from build123d import *

# Parameters (mm, degrees)
F0_W     = 228.6
F0_H     = 101.6
F0_R     = 22.225
F0_R_2   = 3.175
F1_DEPTH = 9.525
F2_DEPTH = 5.08


with BuildPart() as f1:
    # F0 (on Top) → F1 (new body)
    with BuildSketch(Plane.XY):
        with Locations((114.3, -50.8)):
            Rectangle(F0_W, F0_H)
        with Locations((32.385, -69.215)):
            Circle(F0_R, mode=Mode.SUBTRACT)
        with Locations((12.446, -19.05)):
            Circle(F0_R_2, mode=Mode.SUBTRACT)
        with Locations((23.241, -19.05)):
            Circle(F0_R_2, mode=Mode.SUBTRACT)
        with Locations((34.036, -19.05)):
            Circle(F0_R_2, mode=Mode.SUBTRACT)
        with Locations((44.831, -19.05)):
            Circle(F0_R_2, mode=Mode.SUBTRACT)
        with BuildLine():
            ThreePointArc((66.04, -22.86), (69.759744, -13.879744), (78.74, -10.16))
            Line((78.74, -10.16), (205.74, -10.16))
            ThreePointArc((205.74, -10.16), (214.720256, -13.879744), (218.44, -22.86))
            Line((218.44, -22.86), (218.44, -78.74))
            ThreePointArc((218.44, -78.74), (214.720256, -87.720256), (205.74, -91.44))
            Line((205.74, -91.44), (78.74, -91.44))
            ThreePointArc((78.74, -91.44), (69.759744, -87.720256), (66.04, -78.74))
            Line((66.04, -78.74), (66.04, -22.86))
        make_face(mode=Mode.SUBTRACT)
        with BuildLine():
            Line((205.74, -10.16), (78.74, -10.16))
            ThreePointArc((78.74, -10.16), (69.759744, -13.879744), (66.04, -22.86))
            Line((66.04, -22.86), (66.04, -78.74))
            ThreePointArc((66.04, -78.74), (69.759744, -87.720256), (78.74, -91.44))
            Line((78.74, -91.44), (205.74, -91.44))
            ThreePointArc((205.74, -91.44), (214.720256, -87.720256), (218.44, -78.74))
            Line((218.44, -78.74), (218.44, -22.86))
            ThreePointArc((218.44, -22.86), (214.720256, -13.879744), (205.74, -10.16))
        make_face()
    extrude(amount=-F1_DEPTH)

    # F0 (on Top) → F2 (cut)
    with BuildSketch(Plane.XY):
        with BuildLine():
            Line((205.74, -10.16), (78.74, -10.16))
            ThreePointArc((78.74, -10.16), (69.759744, -13.879744), (66.04, -22.86))
            Line((66.04, -22.86), (66.04, -78.74))
            ThreePointArc((66.04, -78.74), (69.759744, -87.720256), (78.74, -91.44))
            Line((78.74, -91.44), (205.74, -91.44))
            ThreePointArc((205.74, -91.44), (214.720256, -87.720256), (218.44, -78.74))
            Line((218.44, -78.74), (218.44, -22.86))
            ThreePointArc((218.44, -22.86), (214.720256, -13.879744), (205.74, -10.16))
        make_face()
    extrude(amount=-F2_DEPTH, mode=Mode.SUBTRACT)


solid = f1.part
For this review, take the finished solid that the model builds, in its own axes (mm). A direction names the side the tool comes from. Give positions to 0.01 mm unless a question says otherwise; leave off trailing zeros. Loops run counter-clockwise (first coordinate to the right, second up) from the corner with the lowest first, then second, coordinate; pieces in that order, holes last.
Item 1: Take a section at D-D, the plane z = -1.5. State the section outline as (x, y) points (3 decimals), and give its area (3 significant figures).
Item 2: Insertion check: pin 1 (4 mm diameter, centred on x = 123.5, y = -67, fed in from +Z); pin 2 (5.5 mm diameter, centred on x = 12.446, y = -19.05, fed in from -Z). Each pin has a flat end and moves straight along its axis. Give the tip position at first contact, or say it passes through.
Item 3: Take a section at B-B, the plane x = 45.5. State the section outline as (y, z) points (3 decimals).
Item 4: For line 1 along X through (y, z) = (-72, -3.75); line 2 along Y through (x, z) = (35, -2.25); line 3 along Y through (x, z) = (185, -4.5), list the stretches that pass through material, from the lowest coordinate up.
Item 5: Tool access review of faces 4 (the flat face through (218.44, -51, -3)), 5 (the flat face through (113, 0, -5)): name each direction out of +Z, -Z, +X, -X, +Y, -Y from which nothing blocks a thin tool from reaching the whole face with its end or side.
Item 6: Take a section at A-A, the plane y = -58. State the section outline as (x, z) points (3 decimals), and give its area (3 significant figures).
Item 7: Draft analysis for pull direction Y (two halves, no side actions). For faces 1 (the flat face through (113, -101.6, -5)), 2 (the flat face through (141, -50, -5.08)), 3 (the flat face through (0, -52, -5)), state which applies: +Y half, -Y half, draft (parallel to the pull), parting line (faces both ways), or undercut.
Item 8: Take a section at C-C, the plane y = -19.05. State the section outline as (x, z) points (3 decimals), and give its area (3 significant figures).
Calculated:
1. outline: (0, -101.6) - (228.6, -101.6) - (228.6, 0) - (0, 0) - close; hole circle Ø6.35 at (12.446, -19.05); hole circle Ø44.45 at (32.385, -69.215); hole circle Ø6.35 at (23.241, -19.05); hole circle Ø6.35 at (34.036, -19.05); hole circle Ø6.35 at (44.831, -19.05); hole (66.04, -78.74) arc R12.7 ccw to (78.74, -91.44) - (205.74, -91.44) arc R12.7 ccw to (218.44, -78.74) - (218.44, -22.86) arc R12.7 ccw to (205.74, -10.16) - (78.74, -10.16) arc R12.7 ccw to (66.04, -22.86) - close
1. area: 9,300 mm2
2. pin 1: stops at z = -5.08
2. pin 2: passes through
3. outline: (-101.6, -9.525) - (-87.158, -9.525) - (-87.158, 0) - (-101.6, 0) - close; (-51.272, -9.525) - (-22.154, -9.525) - (-22.154, 0) - (-51.272, 0) - close; (-15.946, -9.525) - (0, -9.525) - (0, 0) - (-15.946, 0) - close
4. line 1: x = 0 to 10.34, 54.43 to 66.04, 218.44 to 228.6
4. line 2: y = -101.6 to -91.29, -47.14 to -22.08, -16.02 to 0
4. line 3: y = -101.6 to -91.44, -10.16 to 0
5. face 4: +Z
5. face 5: +Z, -Z, +X, -X, +Y
6. outline: (0, -9.525) - (13.197, -9.525) - (13.197, 0) - (0, 0) - close; (51.573, -9.525) - (228.6, -9.525) - (228.6, 0) - (218.44, 0) - (218.44, -5.08) - (66.04, -5.08) - (66.04, 0) - (51.573, 0) - close
6. area: 1,040 mm2
7. face 1: -Y half
7. face 2: undercut
7. face 3: draft
8. outline: (0, -9.525) - (9.271, -9.525) - (9.271, 0) - (0, 0) - close; (15.621, -9.525) - (20.066, -9.525) - (20.066, 0) - (15.621, 0) - close; (26.416, -9.525) - (30.861, -9.525) - (30.861, 0) - (26.416, 0) - close; (37.211, -9.525) - (41.656, -9.525) - (41.656, 0) - (37.211, 0) - close; (48.006, -9.525) - (228.6, -9.525) - (228.6, 0) - (217.855, 0) - (217.855, -5.08) - (66.625, -5.08) - (66.625, 0) - (48.006, 0) - close
8. area: 1,170 mm2
